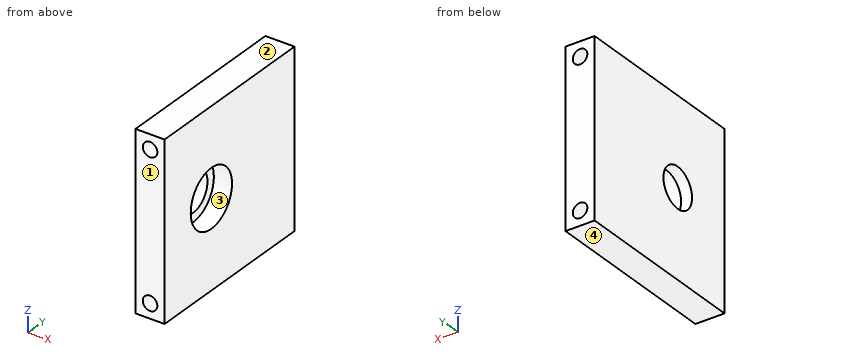
```python
from build123d import *

# Parameters (mm, degrees)
ESQUISSE1_W             = 8
ESQUISSE1_H             = 48
BOSS_EXTRU_1_DEPTH      = 50
ESQUISSE28_R            = 7.95
ENL_V_MAT_EXTRU_1_DEPTH = 10
ESQUISSE29_R            = 8.2
ESQUISSE29_R_2          = 5.5
BOSS_EXTRU_2_DEPTH      = 3
ESQUISSE30_R            = 2
ENL_V_MAT_EXTRU_2_DEPTH = 15
ENL_V_START             = -15
ESQUISSE31_R            = 2
ENL_V_MAT_EXTRU_3_DEPTH = 15


with BuildPart() as part:
    # Esquisse1 → Boss.-Extru.1 (new body)
    with BuildSketch(Plane(origin=(0, 0, 0), x_dir=(1, 0, 0), z_dir=(0, 1, 0))):
        with Locations((4, 24)):
            Rectangle(ESQUISSE1_W, ESQUISSE1_H)
    extrude(amount=BOSS_EXTRU_1_DEPTH)

    # Esquisse28 → Enl_v. mat.-Extru.1 (cut)
    with BuildSketch(Plane(origin=(8, 0, 0), x_dir=(0, 0, -1), z_dir=(1, 0, 0))):
        with Locations((24, 18)):
            Circle(ESQUISSE28_R)
    extrude(amount=-ENL_V_MAT_EXTRU_1_DEPTH, mode=Mode.SUBTRACT)

    # Esquisse29 → Boss.-Extru.2 (add)
    with BuildSketch(Plane.ZY):
        with Locations((-24, 18)):
            Circle(ESQUISSE29_R)
        with Locations((-24, 18)):
            Circle(ESQUISSE29_R_2, mode=Mode.SUBTRACT)
    extrude(amount=-BOSS_EXTRU_2_DEPTH)

    # Esquisse30 → Enl_v. mat.-Extru.2 (cut)
    with BuildSketch(Plane.XZ):
        with Locations(Location((4, -44, 0), (0, 0, 270))):
            Circle(ESQUISSE30_R)
        with Locations(Location((4, -4, 0), (0, 0, 270))):
            Circle(ESQUISSE30_R)
    extrude(amount=-ENL_V_MAT_EXTRU_2_DEPTH, mode=Mode.SUBTRACT)

    # Esquisse31 → Enl_v. mat.-Extru.3 (cut)
    with BuildSketch(Plane(origin=(0, 50, 0), x_dir=(1, 0, 0), z_dir=(0, 1, 0)).offset(ENL_V_START)):
        with Locations(Location((4, 44, 0), (0, 0, 90))):
            Circle(ESQUISSE31_R)
        with Locations(Location((4, 4, 0), (0, 0, 90))):
            Circle(ESQUISSE31_R)
    extrude(amount=ENL_V_MAT_EXTRU_3_DEPTH, mode=Mode.SUBTRACT)


solid = part.part
```
Design review of the part built by this model. Coordinates are the model's own, in mm. Face numbers are marked on the shaded views. Round coordinates to 2 decimals unless told otherwise and drop trailing zeros. Order: outer loops, then holes, each group sorted by start corner. A loop starts at its lowest first (then second) coordinate and runs counter-clockwise, first axis right, second up. Notation, with made-up numbers: (-10, -23.5) - (42, -23.5) arc R15 cw to (42, -3.5) - close; hole circle Ø11 at (31.5, 38.5). An arc over 180 degrees is marked (long way). Return JSON: item names as keys, results as strings.
Q1. Consider section A-A on y = 18. Write out the cut boundary in (x, z), plus the area to 4 significant figures.
Computed values:
{"outline": "(0, -48) - (8, -48) - (8, -31.95) - (3, -31.95) - (3, -29.5) - (0, -29.5) - close; (0, -18.5) - (3, -18.5) - (3, -16.05) - (8, -16.05) - (8, 0) - (0, 0) - close", "area": "271.5 mm2"}
Q2. Consider section C-C on x = 4. Write out the cut boundary in (y, z).
Computed values:
{"outline": "(0, -48) - (50, -48) - (50, -46) - (35, -46) - (35, -42) - (50, -42) - (50, -6) - (35, -6) - (35, -2) - (50, -2) - (50, 0) - (0, 0) - (0, -2) - (15, -2) - (15, -6) - (0, -6) - (0, -42) - (15, -42) - (15, -46) - (0, -46) - close; hole circle Ø15.9 at (18, -24)"}
Q3. Consider section D-D on y = 4. Write out the cut boundary in (x, z).
Computed values:
{"outline": "(0, -48) - (8, -48) - (8, 0) - (0, 0) - close; hole circle Ø4 at (4, -44); hole circle Ø4 at (4, -4)"}
Q4. For pin 1 Ø2 at (x, z) = (3.5, -45) entering from -Y; pin 2 Ø3 at (x, z) = (4, -4) entering from -Y, all flat-tipped, find the tip position at first contact; note any pin that passes through.
Computed values:
{"pin 1": "stops at y = 0", "pin 2": "stops at y = 15"}
Q5. Wall thickness on L1, parallel to Z at x = 4, y = 47; L2, parallel to X at y = 38, z = -44; L3, parallel to Y at x = 6.5, z = -24: over which ranges is each line inside the solid? List them lowest first. Write a range as [from, to].
Computed values:
{"L1": "z = [-48, -46], [-42, -6], [-2, 0]", "L2": "x = [0, 2], [6, 8]", "L3": "y = [0, 10.05], [25.95, 50]"}
Q6. Consider section B-B on z = -24. Write out the cut boundary in (x, y).
Computed values:
{"outline": "(0, 0) - (8, 0) - (8, 10.05) - (3, 10.05) - (3, 12.5) - (0, 12.5) - close; (0, 23.5) - (3, 23.5) - (3, 25.95) - (8, 25.95) - (8, 50) - (0, 50) - close"}
Q7. The part is to be moulded in two halves that separate along Z. For the marked faces 1, 2, 3 and 4, say which applies: pulls with the +Z half, pulls with the -Z half, needs draft (parallel to the pull), parting line crosses it, or undercut.
Computed values:
{"face 1": "needs draft", "face 2": "pulls with the +Z half", "face 3": "undercut", "face 4": "pulls with the -Z half"}
